Autodesk Inventor part; units mm, degrees
ref_plane "YZ Plane" through (0, 0, 0) normal (1, 0, 0) x (0, 1, 0)
ref_plane "XZ Plane" through (0, 0, 0) normal (0, 1, 0) x (-1, 0, 0)
ref_plane "XY Plane" through (0, 0, 0) normal (0, 0, 1) x (1, 0, 0)
sketch "Boceto1" plane through (0, 0, 0) normal (0, 0, 1) x (1, 0, 0)
  line L0 (-20, 0) -> (20, 0)
  line L1 (20, 0) -> (60, 80)
  line L2 (60, 80) -> (60, 120)
  line L3 (60, 120) -> (-60, 120)
  line L4 (-60, 120) -> (-60, 80)
  line L5 (-60, 80) -> (-20, 0)
  circle A0 centre (0, 100) radius 4.15
  circle A1 centre (0, 60) radius 4.15
  circle A2 centre (0, 20) radius 4.15
  circle A3 centre (40, 100) radius 4.15
  circle A4 centre (-40, 100) radius 4.15
  point P0 (0, 0)
  point P1 (0, 0)
  point P2 (0, 120)
  dimension "d0" = 120
  dimension "d1" = 120
  dimension "d2" = 40
  dimension "d3" = 40
  dimension "d4" = 20
  dimension "d5" = 8.3
  dimension "d6" = 40
  dimension "d7" = 40
  dimension "d8" = 40
  dimension "d9" = 40
extrude "Extrusión1" add sketch "Boceto1" along normal blind 6
equation "\"d8\" = d7"
equation "\"d9\" = d7"
properties part number "T"
Read the model definition and answer for the solid it produces. Units are mm, in the model's axes. Coordinates: 2 decimals unless noted, no trailing zeros. Write each loop counter-clockwise with the first axis right and the second up, starting at its lowest first coordinate (ties: lowest second). Pieces come first, ordered by that corner, then holes. Notation, with made-up numbers: (49.5, 62) -> (63.5, 62) arc R22 ccw to (63.5, 79) -> close; hole circle Ø7 at (25.5, 81.25). An arc over 180 degrees is marked (long way). Return JSON: item names as keys, results as strings.
(1) The part is cut by section A-A on y = 20. Give the vertices of the cut face in (x, z), then the cut area to 3 significant figures.
Answers below:
{"outline": "(-30, 0) -> (-4.15, 0) -> (-4.15, 6) -> (-30, 6) -> close; (4.15, 0) -> (30, 0) -> (30, 6) -> (4.15, 6) -> close", "area": "310 mm^2"}
(2) This flat-tipped pin is pushed along its axis until it touches: P1, Ø1, axis at y = 67, z = 1, coming from the +X side. Where does it stop, or does it pass through?
Answers below:
{"P1": "x = 53.75"}
(3) Consider line 1 along Y through (x, z) = (0, 4.7); line 2 along X through (y, z) = (97, 1.5); line 3 along Y through (x, z) = (-40, 1.3). Determine where each line is inside the solid, lowest interval first. Write a range as from..to.
Answers below:
{"line 1": "0..15.85, 24.15..55.85, 64.15..95.85, 104.15..120", "line 2": "-60..-42.87, -37.13..-2.87, 2.87..37.13, 42.87..60", "line 3": "40..95.85, 104.15..120"}
(4) The part is cut by section B-B on x = -40. Give the vertices of the cut face in (y, z).
Answers below:
{"outline": "(40, 0) -> (95.85, 0) -> (95.85, 6) -> (40, 6) -> close; (104.15, 0) -> (120, 0) -> (120, 6) -> (104.15, 6) -> close"}
(5) The part is cut by section D-D on y = 46.5. Give the vertices of the cut face in (x, z), then the cut area to 3 significant figures.
Answers below:
{"outline": "(-43.25, 0) -> (43.25, 0) -> (43.25, 6) -> (-43.25, 6) -> close", "area": "519 mm^2"}
(6) The part is cut by section C-C on z = 3.9. Give the vertices of the cut face in (x, y), then the cut area to 3 significant figures.
Answers below:
{"outline": "(-60, 80) -> (-20, 0) -> (20, 0) -> (60, 80) -> (60, 120) -> (-60, 120) -> close; hole circle Ø8.3 at (-40, 100); hole circle Ø8.3 at (0, 20); hole circle Ø8.3 at (0, 60); hole circle Ø8.3 at (0, 100); hole circle Ø8.3 at (40, 100)", "area": "10,900 mm^2"}
(7) For a pull along Y with two mould halves and no side action, classify faces 1 (the flat face through (-1, 74, 6)), 2 (the cylindrical face through (42.23, 96.5, 2.96)), 3 (the flat face through (-40.3, 40.6, 3)), 4 (the cylindrical face through (-0.54, 55.885, 2.958)) as pulls with the +Y half, pulls with the -Y half, needs draft (parallel to the pull), parting line crosses it, or undercut.
Answers below:
{"face 1": "needs draft", "face 2": "undercut", "face 3": "pulls with the -Y half", "face 4": "undercut"}
